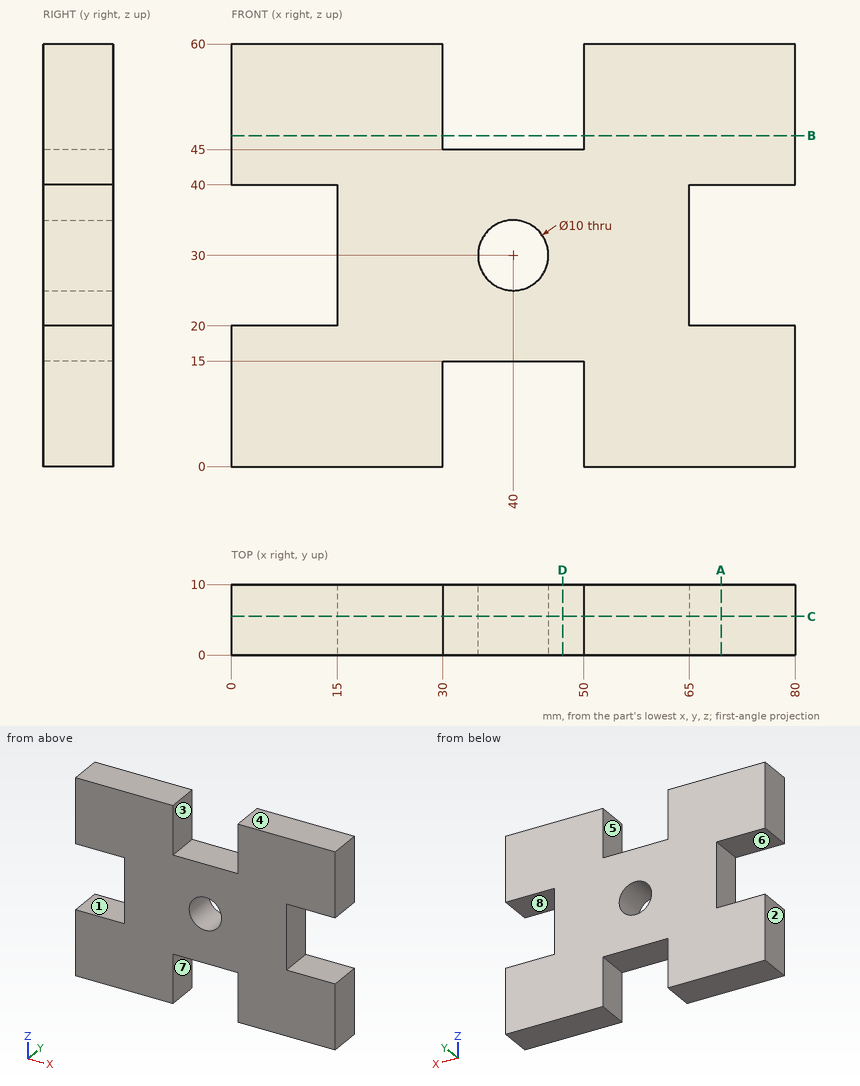
Geometry check sheet. Reference: drawing and pictorial views, mm from the part's lowest x, y, z. A direction names the side the tool comes from. Round coordinates to 2 decimals unless told otherwise and drop trailing zeros. Write each loop counter-clockwise with the first axis right and the second up, starting at its lowest first coordinate (ties: lowest second). Pieces come first, ordered by that corner, then holes. Notation, with made-up numbers: (30, -12.75) -> (40, -12.75) arc R11 ccw to (40, 5.25) -> close; hole circle Ø1 at (89.25, 75.5). An arc over 180 degrees is marked (long way). One line per question, with ' | ' between items. Start each with the question number.
1. Sectioned sample at A-A, the plane x = 69.5. Record the cut outline in (y, z).
2. Depth check by flat-ended pin: pin 1 (6 mm diameter, centred on x = 40, z = 30, fed in from +Y); pin 2 (5 mm diameter, centred on x = 41, y = 7, fed in from -Z); pin 3 (3 mm diameter, centred on y = 4, z = 29, fed in from +X). Enter the tip coordinate at first touch or a pass-through.
3. Sectioned sample at D-D, the plane x = 47. Record the cut outline in (y, z), then the cut area to 3 significant figures.
4. Release check for a two-part mould opening along X. For the marked faces 1, 2 and 3 record: +X half, -X half, draft (parallel to the pull), parting line (faces both ways), or undercut.
5. Scan lines: line 1 along Z through (x, y) = (75.5, 8.5); line 2 along X through (y, z) = (6, 9.5); line 3 along Z through (x, y) = (40, 3.25). Record each from-to range of solid material in increasing order. Write a range as from..to.
6. Sectioned sample at C-C, the plane y = 5.5. Record the cut outline in (x, z).
7. Set-up check for the marked faces 4, 5, 6, 7 and 8: record each of +Z, -Z, +X, -X, +Y, -Y from which the full face is reachable in a straight line by a thin tool's end or side.
8. Sectioned sample at B-B, the plane z = 47. Record the cut outline in (x, y).
Taken from the geometry:
1) outline: (0, 0) -> (10, 0) -> (10, 20) -> (0, 20) -> close; (0, 40) -> (10, 40) -> (10, 60) -> (0, 60) -> close
2) pin 1: passes through | pin 2: stops at z = 15 | pin 3: stops at x = 65
3) outline: (0, 15) -> (10, 15) -> (10, 45) -> (0, 45) -> close | area: 300 mm^2
4) face 1: draft | face 2: -X half | face 3: undercut
5) line 1: z = 0..20, 40..60 | line 2: x = 0..30, 50..80 | line 3: z = 15..25, 35..45
6) outline: (0, 0) -> (30, 0) -> (30, 15) -> (50, 15) -> (50, 0) -> (80, 0) -> (80, 20) -> (65, 20) -> (65, 40) -> (80, 40) -> (80, 60) -> (50, 60) -> (50, 45) -> (30, 45) -> (30, 60) -> (0, 60) -> (0, 40) -> (15, 40) -> (15, 20) -> (0, 20) -> close; hole circle Ø10 at (40, 30)
7) face 4: +Z, +X, -X, +Y, -Y | face 5: +Z, +Y, -Y | face 6: -X, +Y, -Y | face 7: -Z, +Y, -Y | face 8: +X, +Y, -Y
8) outline: (0, 0) -> (30, 0) -> (30, 10) -> (0, 10) -> close; (50, 0) -> (80, 0) -> (80, 10) -> (50, 10) -> close
